CAD build for the part. Positions are in the model's coordinates, mm. Give positions to 0.01 mm unless a question says otherwise; leave off trailing zeros. Loops run counter-clockwise (first coordinate to the right, second up) from the corner with the lowest first, then second, coordinate; pieces in that order, holes last. Notation, with made-up numbers: M 41,-7 L 89,-7 A22 cw 89,7 Z; hole C 36.5,27 d11. An arc over 180 degrees is marked long. Answer as CSV lines item,"result".
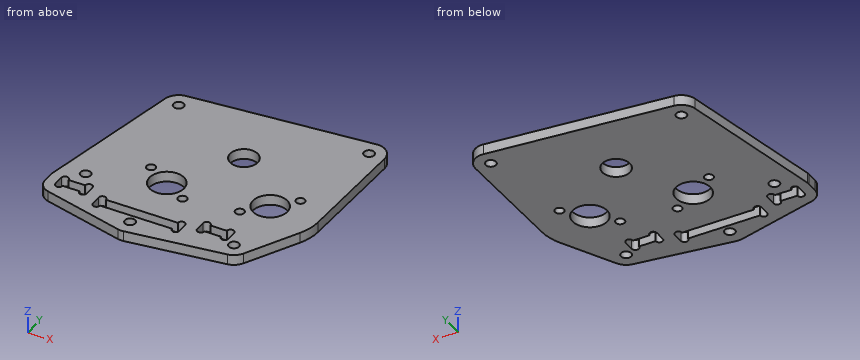
Autodesk Inventor part; units mm, degrees
ref_plane "YZ Plane" through (0, 0, 0) normal (1, 0, 0) x (0, 1, 0)
ref_plane "XZ Plane" through (0, 0, 0) normal (0, 1, 0) x (-1, 0, 0)
ref_plane "XY Plane" through (0, 0, 0) normal (0, 0, 1) x (1, 0, 0)
sketch "スケッチ1" plane through (0, 0, 0) normal (0, 0, 1) x (1, 0, 0)
  circle A0 centre (0, 0) radius 18
  circle A1 centre (-35.3982, 10.7044) radius 1.5
  line L0 (-33.8465, 6.7744) -> (-39.6634, 9.2696)
  arc A2 (-31.9879, 5.2949) -> (-33.8465, 6.7744) centre (-35.6204, 2.6388) ccw
  line L1 (-18.0583, -13.7557) -> (-31.9879, 5.2949)
  arc A3 (-17.339, -17.5569) -> (-18.0583, -13.7557) centre (-21.6908, -16.4118) ccw
  line L2 (-17.339, -17.5569) -> (-23.8868, -42.4405)
  line L3 (21.0739, -11.4259) -> (29.592, -35.7057)
  arc A4 (21.5077, -7.5456) -> (21.0739, -11.4259) centre (25.3202, -9.9362) ccw
  line L4 (34.045, 12.4488) -> (21.5077, -7.5456)
  arc A5 (36.6836, 14.4025) -> (34.045, 12.4488) centre (37.8575, 10.0583) ccw
  line L5 (40.7974, 15.5141) -> (36.6836, 14.4025)
  circle A6 centre (36.7736, 17.5344) radius 1.5
  circle A7 centre (25.6508, -33.5339) radius 1.5
  circle A8 centre (-20.132, -39.9603) radius 1.5
  arc A9 (-23.8868, -42.4405) -> (-19.5065, -44.4166) centre (-20.132, -39.9603) ccw
  line L6 (-19.5065, -44.4166) -> (26.2763, -37.9902)
  arc A10 (26.2763, -37.9902) -> (29.592, -35.7057) centre (25.6508, -33.5339) ccw
  circle A11 centre (27.3908, 10.6821) radius 1.5
  arc A12 (-36.1544, 15.1404) -> (-39.6634, 9.2696) centre (-35.3982, 10.7044) ccw
  arc A13 (40.7942, 15.5132) -> (36.6479, 22.0326) centre (36.7736, 17.5344) ccw
  arc A14 (-0.5868, 20.9918) -> (-3.5285, 20.7014) centre (0, 0) ccw
  line L7 (-36.1544, 15.1404) -> (-3.5285, 20.7014)
  line L8 (-0.5868, 20.9918) -> (36.6479, 22.0326)
  circle A15 centre (14, -17.4118) radius 14 construction
  circle A16 centre (-14, -17.4118) radius 14 construction
  line L9 (-170.6512, -31.4118) -> (202.8656, -31.4118)
  circle A17 centre (-11.0721, -38.6885) radius 3
  circle A18 centre (16.7367, -34.7851) radius 3
  circle A19 centre (26.4774, 17.2466) radius 3
  circle A20 centre (-25.8354, 12.3344) radius 3
  circle A21 centre (0, 0) radius 20.55 construction
  circle A22 centre (-25.8354, 12.3344) radius 1.5
  circle A23 centre (26.4774, 17.2466) radius 1.5
  circle A24 centre (16.7367, -34.7851) radius 1.5
  circle A25 centre (-11.0721, -38.6885) radius 1.5
  circle A26 centre (-11.0721, -38.6885) radius 4.5
  circle A27 centre (16.7367, -34.7851) radius 4.5
  circle A28 centre (26.4774, 17.2466) radius 4.5
  circle A29 centre (-25.8354, 12.3344) radius 4.5
  line L10 (32.7821, 19.6122) -> (19.0889, -6.6924)
  line L11 (-15.7064, -12.7325) -> (-31.5648, 13.0613)
  line L12 (-15.6358, -40.1451) -> (-14.6718, -16.7004)
  line L13 (18.3467, -10.7856) -> (21.1838, -34.078)
  circle A30 centre (0, 0) radius 4
  circle A31 centre (-25.8354, 12.3344) radius 1.5
  circle A32 centre (26.4774, 17.2466) radius 1.5
  circle A33 centre (16.7367, -34.7851) radius 1.5
  circle A34 centre (-11.0721, -38.6885) radius 1.5
  circle A35 centre (14, -17.4118) radius 14 construction
  circle A36 centre (-14, -17.4118) radius 14 construction
  circle A37 centre (0, 0) radius 4
  arc A38 (-26.2561, 16.8147) -> (-29.9839, 14.078) centre (-25.8354, 12.3344) ccw
  arc A39 (30.9006, 16.4185) -> (26.0567, 21.7269) centre (26.4774, 17.2466) ccw
  arc A40 (17.3622, -39.2414) -> (21.1599, -35.6132) centre (16.7367, -34.7851) ccw
  arc A41 (-12.1183, -43.0652) -> (-10.4466, -43.1449) centre (-11.0721, -38.6885) ccw
  circle A42 centre (-14, -17.4118) radius 5
  circle A43 centre (14, -17.4118) radius 5
  circle A44 centre (0, 0) radius 22.3421 construction
  line L14 (-30.3415, -4.2724) -> (0, -28.6685) construction
  line L15 (0, -28.6685) -> (32.9859, -2.1461) construction
  circle A45 centre (-14, -17.4118) radius 8 construction
  circle A46 centre (14, -17.4118) radius 8 construction
  circle A47 centre (-20.2346, -12.3988) radius 1.3
  circle A48 centre (-7.7654, -22.4248) radius 1.3
  circle A49 centre (7.7654, -22.4248) radius 1.3
  circle A50 centre (20.2346, -12.3988) radius 1.3
  line L16 (-170.6512, -31.4118) -> (202.8656, -31.4118)
  line L17 (-42.4, -28.4118) -> (-37.6, -28.4118)
  line L18 (-35.5, -28.4118) -> (-35.5, -31.4118)
  line L19 (-37.6, -31.4118) -> (-42.4, -31.4118)
  line L20 (-44.5, -31.4118) -> (-44.5, -28.4118)
  line L21 (-2.4, -28.4118) -> (2.4, -28.4118)
  line L22 (4.5, -28.4118) -> (4.5, -31.4118)
  line L23 (2.4, -31.4118) -> (-2.4, -31.4118)
  line L24 (-4.5, -31.4118) -> (-4.5, -28.4118)
  line L25 (-30.4, -31.4118) -> (-9.6, -31.4118)
  line L26 (-7.5, -31.4118) -> (-7.5, -34.4118)
  line L27 (-9.6, -34.4118) -> (-30.4, -34.4118)
  line L28 (-32.5, -34.4118) -> (-32.5, -31.4118)
  arc A51 (-42.4, -28.4118) -> (-44.5, -28.4118) centre (-43.45, -28.4118) ccw
  arc A52 (-35.5, -28.4118) -> (-37.6, -28.4118) centre (-36.55, -28.4118) ccw
  arc A53 (-44.5, -31.4118) -> (-42.4, -31.4118) centre (-43.45, -31.4118) ccw
  arc A54 (-37.6, -31.4118) -> (-35.5, -31.4118) centre (-36.55, -31.4118) ccw
  arc A55 (-30.4, -31.4118) -> (-32.5, -31.4118) centre (-31.45, -31.4118) ccw
  arc A56 (-32.5, -34.4118) -> (-30.4, -34.4118) centre (-31.45, -34.4118) ccw
  arc A57 (-7.5, -31.4118) -> (-9.6, -31.4118) centre (-8.55, -31.4118) ccw
  arc A58 (-9.6, -34.4118) -> (-7.5, -34.4118) centre (-8.55, -34.4118) ccw
  arc A59 (-4.5, -31.4118) -> (-2.4, -31.4118) centre (-3.45, -31.4118) ccw
  arc A60 (-2.4, -28.4118) -> (-4.5, -28.4118) centre (-3.45, -28.4118) ccw
  arc A61 (4.5, -28.4118) -> (2.4, -28.4118) centre (3.45, -28.4118) ccw
  arc A62 (2.4, -31.4118) -> (4.5, -31.4118) centre (3.45, -31.4118) ccw
  circle A63 centre (-40, -23.9118) radius 1.5
  circle A64 centre (-40, -23.9118) radius 4.5 construction
  arc A65 (-35.5, -24.5003) -> (-35.5374, -24.4904) centre (-36.55, -28.4118) ccw
  line L29 (-47.5, -28.4118) -> (-47.5, -31.4118)
  arc A66 (-47.5, -31.4118) -> (-44.3916, -35.3508) centre (-43.45, -31.4118) ccw
  line L30 (-47.1836, -26.8425) -> (-29.9839, 14.078)
  line L31 (-26.2561, 16.8147) -> (26.0567, 21.7269)
  line L32 (30.9006, 16.4185) -> (21.1599, -35.6132)
  line L33 (17.3622, -39.2414) -> (-10.4466, -43.1449)
  line L34 (-44.3916, -35.3508) -> (-12.1183, -43.0652)
  arc A67 (-47.1836, -26.8425) -> (-47.5, -28.4118) centre (-43.45, -28.4118) ccw
  circle A68 centre (-11.4931, -19.1593) radius 4
  circle A69 centre (16.245, -15.3385) radius 4
  dimension "d74" = 9
  dimension "d0" = 36
  dimension "d1" = 9
  dimension "d2" = 9
  dimension "d3" = 3
  dimension "d4" = 6
  dimension "d5" = 6
  dimension "d6" = 6
  dimension "d7" = 6
  dimension "d8" = 3
  dimension "d9" = 3
  dimension "d10" = 3
  dimension "d11" = 3
  dimension "d12" = 9
  dimension "d13" = 9
  dimension "d14" = 9
  dimension "d15" = 9
  dimension "d16" = 8
  dimension "d50" = 3
  dimension "d51" = 3
  dimension "d52" = 3
  dimension "d53" = 3
  dimension "d54" = 10
  dimension "d55" = 10
  dimension "d56" = 3
  dimension "d57" = 3
  dimension "d58" = 2.6
  dimension "d59" = 2.6
  dimension "d60" = 2.6
  dimension "d61" = 2.6
  dimension "d62" = 9
  dimension "d63" = 3
  dimension "d64" = 9
  dimension "d65" = 3
  dimension "d66" = 4.5
  dimension "d67" = 40
  dimension "d68" = 25
  dimension "d69" = 3
  dimension "d70" = 3
  dimension "d71" = 3
  dimension "d72" = 2.1
  dimension "d73" = 3
  dimension "d75" = 4.5
  dimension "d76" = 3
  dimension "d77" = 3
  dimension "d78" = 4.05
sketch "スケッチ2" plane through (0, 0, 0) normal (0, 0, 1) x (1, 0, 0)
  circle A0 centre (-25.8354, 12.3344) radius 1.5
  circle A1 centre (26.4774, 17.2466) radius 1.5
  circle A2 centre (16.7367, -34.7851) radius 1.5
  circle A3 centre (-11.0721, -38.6885) radius 1.5
  circle A4 centre (14, -17.4118) radius 14 construction
  circle A5 centre (-14, -17.4118) radius 14 construction
  circle A6 centre (0, 0) radius 4
  arc A7 (-26.2561, 16.8147) -> (-30.2492, 13.2111) centre (-25.8354, 12.3344) ccw
  arc A8 (30.9763, 17.1458) -> (26.0567, 21.7269) centre (26.4774, 17.2466) ccw
  arc A9 (17.3622, -39.2414) -> (20.7179, -36.8828) centre (16.7367, -34.7851) ccw
  arc A10 (-12.177, -43.0508) -> (-10.4466, -43.1449) centre (-11.0721, -38.6885) ccw
  circle A11 centre (-14, -17.4118) radius 5
  circle A12 centre (14, -17.4118) radius 5
  circle A13 centre (0, 0) radius 22.3421 construction
  line L0 (-30.3415, -4.2724) -> (0, -28.6685) construction
  line L1 (0, -28.6685) -> (32.9859, -2.1461) construction
  circle A14 centre (-14, -17.4118) radius 8 construction
  circle A15 centre (14, -17.4118) radius 8 construction
  circle A16 centre (-20.2346, -12.3988) radius 1.3
  circle A17 centre (-7.7654, -22.4248) radius 1.3
  circle A18 centre (7.7654, -22.4248) radius 1.3
  circle A19 centre (20.2346, -12.3988) radius 1.3
  line L2 (-33.6846, -30.1593) -> (-28.8846, -30.1593)
  line L3 (-26.7846, -30.1593) -> (-26.7846, -33.1593)
  line L4 (-28.8846, -33.1593) -> (-33.6846, -33.1593)
  line L5 (-35.7846, -33.1593) -> (-35.7846, -30.1593)
  line L6 (7.3154, -30.1593) -> (12.1154, -30.1593)
  line L7 (14.2154, -30.1593) -> (14.2154, -33.1593)
  line L8 (12.1154, -33.1593) -> (7.3154, -33.1593)
  line L9 (5.2154, -33.1593) -> (5.2154, -30.1593)
  line L10 (-21.1846, -33.1593) -> (-0.3846, -33.1593)
  line L11 (1.7154, -33.1593) -> (1.7154, -36.1593)
  line L12 (-0.3846, -36.1593) -> (-21.1846, -36.1593)
  line L13 (-23.2846, -36.1593) -> (-23.2846, -33.1593)
  arc A20 (-33.6846, -30.1593) -> (-35.7846, -30.1593) centre (-34.7346, -30.1593) ccw
  arc A21 (-26.7846, -30.1593) -> (-28.8846, -30.1593) centre (-27.8346, -30.1593) ccw
  arc A22 (-35.7846, -33.1593) -> (-33.6846, -33.1593) centre (-34.7346, -33.1593) ccw
  arc A23 (-28.8846, -33.1593) -> (-26.7846, -33.1593) centre (-27.8346, -33.1593) ccw
  arc A24 (-21.1846, -33.1593) -> (-23.2846, -33.1593) centre (-22.2346, -33.1593) ccw
  arc A25 (-23.2846, -36.1593) -> (-21.1846, -36.1593) centre (-22.2346, -36.1593) ccw
  arc A26 (1.7154, -33.1593) -> (-0.3846, -33.1593) centre (0.6654, -33.1593) ccw
  arc A27 (-0.3846, -36.1593) -> (1.7154, -36.1593) centre (0.6654, -36.1593) ccw
  arc A28 (5.2154, -33.1593) -> (7.3154, -33.1593) centre (6.2654, -33.1593) ccw
  arc A29 (7.3154, -30.1593) -> (5.2154, -30.1593) centre (6.2654, -30.1593) ccw
  arc A30 (14.2154, -30.1593) -> (12.1154, -30.1593) centre (13.1654, -30.1593) ccw
  arc A31 (12.1154, -33.1593) -> (14.2154, -33.1593) centre (13.1654, -33.1593) ccw
  circle A32 centre (-31.2846, -25.6593) radius 1.5
  circle A33 centre (-31.2846, -25.6593) radius 4.5 construction
  line L14 (-38.7846, -30.1593) -> (-38.7846, -33.1593)
  arc A34 (-38.7846, -33.1593) -> (-35.729, -37.0854) centre (-34.7346, -33.1593) ccw
  line L15 (-38.707, -29.3703) -> (-30.2492, 13.2111)
  line L16 (-26.2561, 16.8147) -> (26.0567, 21.7269)
  line L17 (17.3622, -39.2414) -> (-10.4466, -43.1449)
  line L18 (-35.729, -37.0854) -> (-12.177, -43.0508)
  arc A35 (-38.707, -29.3703) -> (-38.7846, -30.1593) centre (-34.7346, -30.1593) ccw
  circle A36 centre (-11.4931, -19.1593) radius 4 construction
  circle A37 centre (16.245, -15.3385) radius 4 construction
  circle A38 centre (-11.4931, -19.1593) radius 5
  circle A39 centre (16.245, -15.3385) radius 5
  line L19 (-26.4603, -10.181) -> (3.9121, -28.4004) construction
  line L20 (3.9121, -28.4004) -> (26.0888, -4.913) construction
  circle A40 centre (-11.4931, -19.1593) radius 8 construction
  circle A41 centre (16.245, -15.3385) radius 8 construction
  circle A42 centre (-18.3534, -15.044) radius 1.3
  circle A43 centre (-4.6327, -23.2746) radius 1.3
  circle A44 centre (10.7528, -21.1553) radius 1.3
  circle A45 centre (21.7373, -9.5217) radius 1.3
  circle A46 centre (-11.4931, -19.1593) radius 14
  arc A47 (28.6309, -21.8646) -> (30.2415, -15.6521) centre (16.245, -15.3385) ccw
  circle A48 centre (16.7367, -34.7851) radius 3
  line L21 (30.9763, 17.1458) -> (30.2415, -15.6521)
  line L22 (28.6309, -21.8646) -> (20.7179, -36.8828)
  circle A49 centre (-11.0721, -38.6885) radius 3
  dimension "d91" = 6
  dimension "d17" = 3
  dimension "d18" = 3
  dimension "d19" = 3
  dimension "d20" = 3
  dimension "d21" = 10
  dimension "d22" = 10
  dimension "d23" = 3
  dimension "d24" = 3
  dimension "d25" = 2.6
  dimension "d26" = 2.6
  dimension "d27" = 2.6
  dimension "d28" = 2.6
  dimension "d29" = 9
  dimension "d30" = 3
  dimension "d31" = 9
  dimension "d32" = 3
  dimension "d35" = 25
  dimension "d36" = 3
  dimension "d37" = 3.5
  dimension "d38" = 3.5
  dimension "d39" = 2.1
  dimension "d40" = 3
  dimension "d42" = 9
  dimension "d44" = 4.5
  dimension "d45" = 3
  dimension "d46" = 3
  dimension "d47" = 4.05
  dimension "d79" = 10
  dimension "d80" = 10
  dimension "d81" = 3
  dimension "d82" = 3
  dimension "d83" = 2.6
  dimension "d84" = 2.6
  dimension "d85" = 2.6
  dimension "d86" = 2.6
  dimension "d89" = 28
  dimension "d90" = 28
  dimension "d92" = 50
  dimension "d93" = 6
extrude "押し出し1" add sketch "スケッチ2" along normal blind 3 contours L16 A8 L21 A47 L22 A9 L17 A10 L18 A34 L14 A35 L15 A7 | A11 A38 | A11 A38 A17 | A38 A11 A42 | A42 A11 | A11 A42 | A38 A17 | A17 A38 | A12 A39 | A12 A39 A19 | A39 A12 A44 | A44 A12 | A12 A44 | A39 A19 | A19 A39 | A16 | A18 | A48 A31 | A46 | L12 A49 | A43 | A45 picked at (19.1924, -35.1468) picked at (-11.0118, -36.506)
extrude "押し出し2" cut sketch "スケッチ2" along normal blind 10 contours A11 A38 | A11 A38 A17 | A42 A11 | A11 A42 | A17 A38 | A12 A39 | A12 A39 A19 | A44 A12 | A12 A44 | A39 A19 | A43 | A45 picked at (-8.0787, -22.1504) picked at (19.8993, -12.6458)
equation "\"d71\" = d70"
equation "\"d38\" = d37"
properties part number "脚モーターマウント" material "アルミニウム 2014-T4"
1) Flat gauge pins, fed straight in: pin 1 (0.9 mm diameter, centred on x = -7, z = 1, fed in from -Y); pin 2 (2.5 mm diameter, centred on x = -25.84, y = 12.33, fed in from +Z); pin 3 (1.5 mm diameter, centred on y = -15, z = 0.5, fed in from -X); pin 4 (1.5 mm diameter, centred on y = -31.5, z = 1.5, fed in from +X). Where does each tip first touch, or does it go through?
Answer below:
pin 1,"stops at y = -42.72"
pin 2,"passes through"
pin 3,"stops at x = -36"
pin 4,"stops at x = 23.95"
2) Band-saw the part on A-A on y = -12.5. Give the cut face in (x, z), and give its area (3 significant figures).
Answer below:
outline,"M -35.36,0 L 12.13,0 L 12.13,3 L -35.36,3 Z; M 20.36,0 L 30.31,0 L 30.31,3 L 20.36,3 Z"
area,"172 mm^2"
3) Band-saw the part on C-C on x = 8.5. Give the cut face in (y, z).
Answer below:
outline,"M -40.49,0 L -33.16,0 L -33.16,3 L -40.49,3 Z; M -30.16,0 L 20.08,0 L 20.08,3 L -30.16,3 Z"
4) Band-saw the part on D-D on z = 0.8. Give the number of separate pieces and of enclosed holes in the cut face, and give its area (3 significant figures).
Answer below:
separate pieces,"1"
enclosed holes,"15"
area,"3,360 mm^2"
5) Band-saw the part on B-B on x = 0.5. Give the cut face in (y, z), and give its area (3 significant figures).
Answer below:
outline,"M -41.61,0 L -37.2,0 L -37.2,3 L -41.61,3 Z; M -32.12,0 L -3.97,0 L -3.97,3 L -32.12,3 Z; M 3.97,0 L 19.33,0 L 19.33,3 L 3.97,3 Z"
area,"144 mm^2"
6) Drill centre lines: line 1 (Y direction, x = 0, z = 1.2); line 2 (X direction, y = -20.5, z = 1.4); line 3 (X direction, y = -35, z = 2.65). Where is each one in solid material? Low to high. Write a range as from..to.
Answer below:
line 1,"y = -41.68..-36.97, -32.35..-4, 4..19.28"
line 2,"x = -36.95..-16.31, -6.68..9.63, 11.88..29.26"
line 3,"x = -38.34..-23.28, 1.72..15.25, 18.22..21.71"
